Autodesk Inventor part; units mm, degrees
ref_plane "YZ Plane" through (0, 0, 0) normal (1, 0, 0) x (0, 1, 0)
ref_plane "XZ Plane" through (0, 0, 0) normal (0, 1, 0) x (-1, 0, 0)
ref_plane "XY Plane" through (0, 0, 0) normal (0, 0, 1) x (1, 0, 0)
sketch "Sketch1" plane through (0, 0, 0) normal (0, 0, 1) x (1, 0, 0)
  line L0 (0, 0) -> (-167.5654, 0)
  line L1 (-167.5654, 0) -> (-167.5654, -1490)
  line L2 (-167.5654, -1490) -> (0, -1490)
  line L3 (0, -1490) -> (0, 0)
  line L4 (-167.5654, -1390) -> (-66, -1390)
  line L5 (-66, -1390) -> (-66, -1385)
  line L6 (-66, -1385) -> (-167.5654, -1385)
  line L7 (-167.5654, -1385) -> (-167.5654, -1390)
  line L8 (-167.5654, -890) -> (-66, -890)
  line L9 (-66, -890) -> (-66, -885)
  line L10 (-66, -885) -> (-167.5654, -885)
  line L11 (-167.5654, -885) -> (-167.5654, -890)
  line L12 (-167.5654, -390) -> (-66, -390)
  line L13 (-66, -390) -> (-66, -385)
  line L14 (-66, -385) -> (-167.5654, -385)
  line L15 (-167.5654, -385) -> (-167.5654, -390)
  circle A0 centre (-167.5654, -155) radius 30
  point P0 (-167.5654, -385)
  point P1 (-167.5654, -390)
  point P2 (-167.5654, -885)
  point P3 (-167.5654, -890)
  point P4 (-167.5654, -125)
  point P5 (-167.5654, -185)
  dimension "d0" = 1490
  dimension "d1" = 167.5654
  dimension "d2" = 5
  dimension "d4" = 100
  dimension "d7" = 500
  dimension "d23" = 66
  dimension "d28" = 60
  dimension "d29" = 1335
extrude "Plate1" add sketch "Sketch1" along normal blind 4 contours L3 L2 L1 L4 L5 L6 L8 L9 L10 L12 L13 L14 A0 L0
sketch "Sketch2" plane through (-4, 0, 0) normal (1, 0, 0) x (0, 1, 0)
  line L0 (-1490, 0) -> (0, 0)
  line L1 (0, 0) -> (0, 60)
  line L2 (0, 60) -> (-1490, 60)
  line L3 (-1490, 60) -> (-1490, 0)
edge flange "Flange1" height 60 angle 90 thickness 4 bend radius 4 thickness toward (1, 0, 0) relief tear relief width 4 relief depth 2 edges at (0, -745, 4) wall of the first edge with corners at (-4, -1490, 0) (-4, 0, 0) (-4, 0, 60) (-4, -1490, 60)
bend "Bend1"
corner "Corner1"
chamfer "Corner Chamfer1" distance 3 angle 45 6 edges at (-167.5654, -1390, 2) (-167.5654, -1385, 2) (-167.5654, -890, 2) (-167.5654, -885, 2) (-167.5654, -385, 2) (-167.5654, -390, 2)
equation "\"d0\" = Стрингер_длина"
equation "\"d1\" = стрингер_глубина_3"
equation "\"d2\" = паз_под_стрингер_толщина"
equation "\"d23\" = паз_под_стрингер_глубина - Thickness"
equation "\"d28\" = 2 * радиус_выреза_под_сварку"
equation "\"d12\" = Thickness"
equation "\"d13\" = BendReliefWidth"
equation "\"d14\" = BendReliefDepth"
equation "\"d15\" = MinimumRemnant"
equation "\"d16\" = TransitionRadius"
equation "\"d17\" = ребро_усилителей"
equation "\"d19\" = BendRadius"
equation "\"d20\" = CornerReliefSize"
equation "\"d21\" = GapSize"
equation "\"d22\" = JacobiRadiusSize"
equation "\"BendRadius\" = Thickness"
equation "\"BendReliefWidth\" = Thickness"
equation "\"BendReliefDepth\" = 0.5 * Thickness"
equation "\"CornerReliefSize\" = 4 * Thickness"
equation "\"MinimumRemnant\" = 2 * Thickness"
equation "\"TransitionRadius\" = BendRadius"
equation "\"JacobiRadiusSize\" = BendRadius"
equation "\"GapSize\" = Thickness"
properties part number "0236 GBK stringer 3" material "Steel"
Read the model definition and answer for the solid it produces. Units are mm, in the model's axes. A direction names the side the tool comes from. Give positions to 0.01 mm unless a question says otherwise; leave off trailing zeros. Order: outer loops, then holes, each group sorted by start corner. A loop starts at its lowest first (then second) coordinate and runs counter-clockwise, first axis right, second up. Notation, with made-up numbers: (63, 9.5) -> (92, 9.5) arc R16 ccw to (92, 21.5) -> close; hole circle Ø11 at (-27, 51). An arc over 180 degrees is marked (long way). Write item = value, one per line.
1. Straight lines are drawn through the part: line 1 along Z through (x, y) = (-83.5, -968); line 2 along X through (y, z) = (-1100, 25). For each, find the intervals that lie inside material, in ascending order.
Numbers:
line_1 = 0 to 4
line_2 = -4 to 0
2. A cutting plane is placed at A-A, the plane x = -113. Write down the section's boundary in (y, z), and give its area (3 significant figures).
Numbers:
outline = (-1490, 0) -> (-1390, 0) -> (-1390, 4) -> (-1490, 4) -> close; (-1385, 0) -> (-890, 0) -> (-890, 4) -> (-1385, 4) -> close; (-885, 0) -> (-390, 0) -> (-390, 4) -> (-885, 4) -> close; (-385, 0) -> (0, 0) -> (0, 4) -> (-385, 4) -> close
area = 5,900 mm²
3. A cutting plane is placed at C-C, the plane z = 27. Write down the section's boundary in (x, y), and give its area (3 significant figures).
Numbers:
outline = (-4, -1490) -> (0, -1490) -> (0, 0) -> (-4, 0) -> close
area = 5,960 mm²
4. A cutting plane is placed at B-B, the plane y = -1041. Write down the section's boundary in (x, z).
Numbers:
outline = (-167.57, 0) -> (-8, 0) arc R8 ccw to (0, 8) -> (0, 60) -> (-4, 60) -> (-4, 8) arc R4 cw to (-8, 4) -> (-167.57, 4) -> close
5. The mould has two halves that part along Y. Classify faces 1 (the face through (-137.573, -154.34, 1.972)), 2 (the face through (-59, -1490, 3)), 3 (the face through (-89, -735, 0)): +Y half, -Y half, draft (parallel to the pull), parting line (faces both ways), or undercut.
Numbers:
face_1 = undercut
face_2 = -Y half
face_3 = draft
6. For faces 4 (the face through (-59, 0, 3)), 5 (the face through (-89, -735, 4)), determine the directions among +Z, -Z, +X, -X, +Y, -Y from which every point of the face is accessible in a straight line to the end or side of a thin tool.
Numbers:
face_4 = +Z, -Z, +X, -X, +Y
face_5 = +Z, -X, +Y, -Y
7. A cutting plane is placed at D-D, the plane x = -28. Write down the section's boundary in (y, z), and give its area (3 significant figures).
Numbers:
outline = (-1490, 0) -> (0, 0) -> (0, 4) -> (-1490, 4) -> close
area = 5,960 mm²
8. Given pin 1 (1.2 mm diameter, centred on y = -888, z = 2.5, fed in from -X); pin 2 (12 mm diameter, centred on x = -135, y = -640.5, fed in from +Z); pin 3 (1 mm diameter, centred on y = -998.5, z = 21, fed in from +X); pin 4 (5 mm diameter, centred on y = -1182.5, z = 51.5, fed in from -X), each flat-ended and moving along its own axis, determine where each tip first touches the part or whether it passes through.
Numbers:
pin_1 = -66
pin_2 = 4
pin_3 = 0
pin_4 = -4
